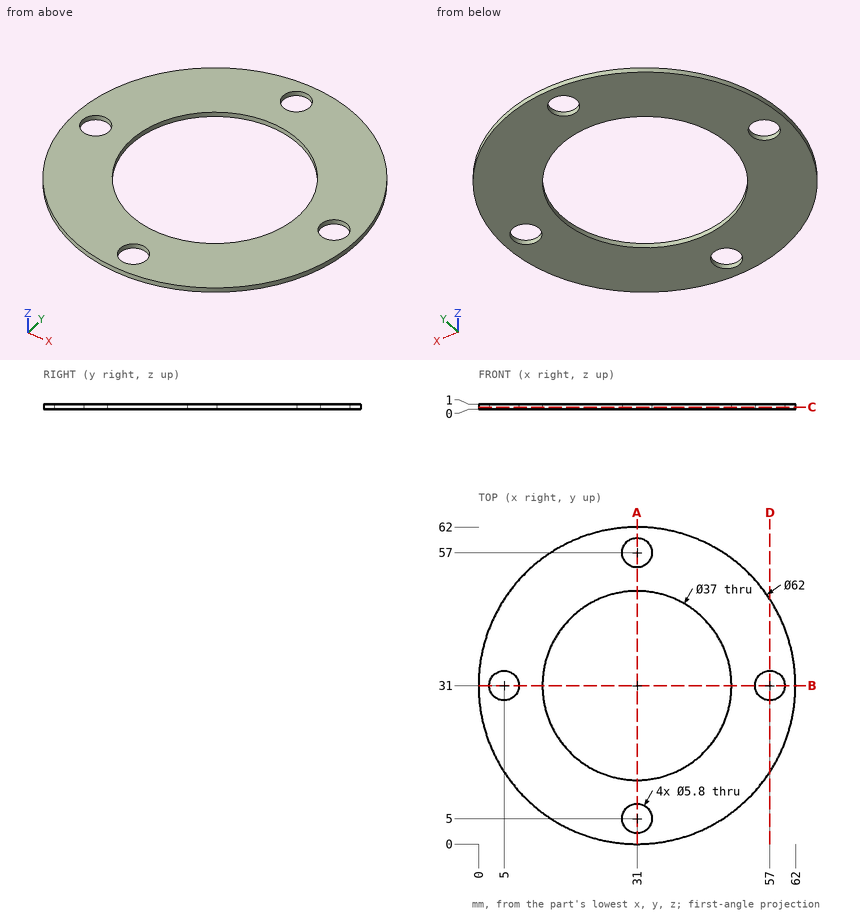
Study the drawing (mm; zero at the part's minimum x, y, z) and answer. Coordinates: 2 decimals unless noted, no trailing zeros. Write each loop counter-clockwise with the first axis right and the second up, starting at its lowest first coordinate (ties: lowest second). Pieces come first, ordered by that corner, then holes. Notation, with made-up numbers: M -30.75,71.25 L 0.25,71.25 A15 ccw 0.25,75.25 Z; hole C 24.5,52 d4. An arc over 180 degrees is marked long. Use a Markdown table: item, result. Add a question column.
1. Section C-C (z = 0.4) is taken. Give the vertices of the cut face in (x, y), plus the area to 3 significant figures.
2. Section D-D (x = 57) is taken. Give the vertices of the cut face in (y, z).
3. Straight lines are drawn through the part: line 1 along Y through (x, z) = (31, 0.55); line 2 along Y through (x, z) = (15.5, 0.15); line 3 along Y through (x, z) = (44.5, 0.35). For each, find the intervals that lie inside material, in ascending order. Write a range as [from, to].
4. Given P1, Ø3.5, axis at x = 57, y = 31, coming from the +Z side, flat-ended and moving along its own axis, determine where the tip first touches the part or whether it passes through.
5. Section A-A (x = 31) is taken. Give the vertices of the cut face in (y, z).
Data:
| question | item | result |
|---|---|---|
| 1 | outline | C 31,31 d62; hole C 5,31 d5.8; hole C 31,31 d37; hole C 31,5 d5.8; hole C 31,57 d5.8; hole C 57,31 d5.8 |
| 1 | area | 1,840 mm2 |
| 2 | outline | M 14.12,0 L 28.1,0 L 28.1,1 L 14.12,1 Z; M 33.9,0 L 47.88,0 L 47.88,1 L 33.9,1 Z |
| 3 | line 1 | y = [0, 2.1], [7.9, 12.5], [49.5, 54.1], [59.9, 62] |
| 3 | line 2 | y = [4.15, 20.9], [41.1, 57.85] |
| 3 | line 3 | y = [3.09, 18.35], [43.65, 58.91] |
| 4 | P1 | passes through |
| 5 | outline | M 0,0 L 2.1,0 L 2.1,1 L 0,1 Z; M 7.9,0 L 12.5,0 L 12.5,1 L 7.9,1 Z; M 49.5,0 L 54.1,0 L 54.1,1 L 49.5,1 Z; M 59.9,0 L 62,0 L 62,1 L 59.9,1 Z |
